Geometry check sheet. Reference: the model listing, model coordinates, mm. Give positions to 0.01 mm unless a question says otherwise; leave off trailing zeros. Write each loop counter-clockwise with the first axis right and the second up, starting at its lowest first coordinate (ties: lowest second). Pieces come first, ordered by that corner, then holes. Notation, with made-up numbers: (29, 42.25) - (76, 42.25) arc R24 ccw to (76, 78.25) - close; hole circle Ø2 at (-17, 80.5). An arc over 180 degrees is marked (long way). Use a Markdown table: item, result.
```python
from build123d import *

# Parameters (mm, degrees)
F1_DEPTH = 1.6
F2_DEPTH = 5


with BuildPart() as f1:
    # F0 (on Top) → F1 (new body)
    with BuildSketch(Plane.XY):
        with BuildLine():
            Line((51, 62), (-38, 62))
            ThreePointArc((-38, 62), (-47.192388, 58.192388), (-51, 49))
            Line((-51, 49), (-51, -49))
            ThreePointArc((-51, -49), (-47.192388, -58.192388), (-38, -62))
            Line((-38, -62), (51, -62))
            Line((51, -62), (51, -56))
            Line((51, -56), (-38, -56))
            ThreePointArc((-38, -56), (-42.949747, -53.949747), (-45, -49))
            Line((-45, -49), (-45, 49))
            ThreePointArc((-45, 49), (-42.949747, 53.949747), (-38, 56))
            Line((-38, 56), (51, 56))
            Line((51, 56), (51, 62))
        make_face()
    extrude(amount=F1_DEPTH)

    # F0 (on Top) → F2 (join)
    with BuildSketch(Plane.XY):
        with BuildLine():
            ThreePointArc((-51, 49), (-47.192388, 58.192388), (-38, 62))
            Line((-38, 62), (51, 62))
            Line((51, 62), (51, 64))
            Line((51, 64), (-38, 64))
            ThreePointArc((-38, 64), (-48.606602, 59.606602), (-53, 49))
            Line((-53, 49), (-53, -49))
            ThreePointArc((-53, -49), (-48.606602, -59.606602), (-38, -64))
            Line((-38, -64), (51, -64))
            Line((51, -64), (51, -62))
            Line((51, -62), (-38, -62))
            ThreePointArc((-38, -62), (-47.192388, -58.192388), (-51, -49))
            Line((-51, -49), (-51, 49))
        make_face()
    extrude(amount=F2_DEPTH)


solid = f1.part
```
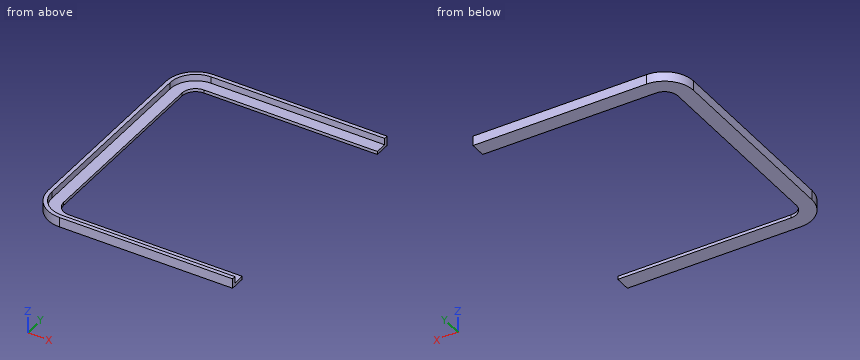
1) Material ranges on L1, parallel to Y at x = -33.5, z = 3.15; L2, parallel to Y at x = 41, z = 0.7; L3, parallel to X at y = 33.5, z = 1.25, recorded low to high. Write a range as from..to.
Working result:
| item | result |
|---|---|
| L1 | y = -64..-62, 62..64 |
| L2 | y = -64..-56, 56..64 |
| L3 | x = -53..-45 |
2) Depth check by flat-ended pin: P1, Ø1.7, axis at y = 20, z = 4, coming from the +X side; P2, Ø1.8, axis at y = 12, z = 1, coming from the +X side. Enter the tip coordinate at first touch or a pass-through.
Working result:
| item | result |
|---|---|
| P1 | stops at x = -51 |
| P2 | stops at x = -45 |
3) Section check D-D on y = -53. Record the boundary of the cut face in (x, z), then the cut area to 3 significant figures.
Working result:
| item | result |
|---|---|
| outline | (-52.46, 0) - (-43.74, 0) - (-43.74, 1.6) - (-50.37, 1.6) - (-50.37, 5) - (-52.46, 5) - close |
| area | 21.0 mm² |
4) Section check A-A on z = 2.9. Record the boundary of the cut face in (x, y), then the cut area to 3 significant figures.
Working result:
| item | result |
|---|---|
| outline | (-53, -49) arc R15 ccw to (-38, -64) - (51, -64) - (51, -62) - (-38, -62) arc R13 cw to (-51, -49) - (-51, 49) arc R13 cw to (-38, 62) - (51, 62) - (51, 64) - (-38, 64) arc R15 ccw to (-53, 49) - close |
| area | 640 mm² |
5) Section check B-B on x = 23.5. Record the boundary of the cut face in (y, z).
Working result:
| item | result |
|---|---|
| outline | (-64, 0) - (-56, 0) - (-56, 1.6) - (-62, 1.6) - (-62, 5) - (-64, 5) - close; (56, 0) - (64, 0) - (64, 5) - (62, 5) - (62, 1.6) - (56, 1.6) - close |
6) Section check C-C on y = 1.5. Record the boundary of the cut face in (x, z).
Working result:
| item | result |
|---|---|
| outline | (-53, 0) - (-45, 0) - (-45, 1.6) - (-51, 1.6) - (-51, 5) - (-53, 5) - close |
